The model under review builds one solid part; all positions refer to its coordinate system, in mm. Round coordinates to 2 decimals unless told otherwise and drop trailing zeros. Order: outer loops, then holes, each group sorted by start corner. A loop starts at its lowest first (then second) coordinate and runs counter-clockwise, first axis right, second up.
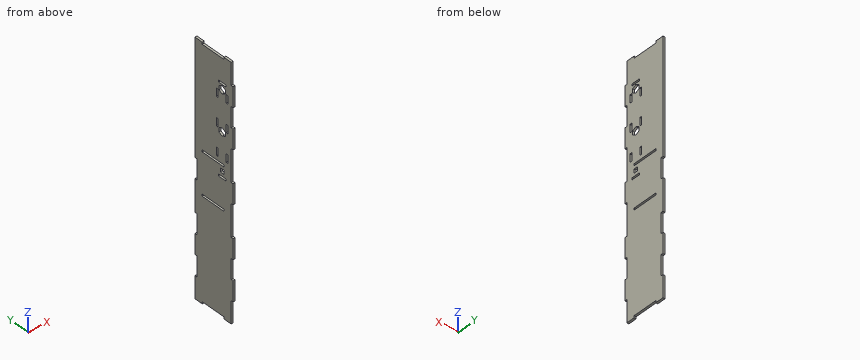
Autodesk Inventor part; units mm, degrees
ref_plane "YZ Plane" through (0, 0, 0) normal (1, 0, 0) x (0, 1, 0)
ref_plane "XZ Plane" through (0, 0, 0) normal (0, 1, 0) x (-1, 0, 0)
ref_plane "XY Plane" through (0, 0, 0) normal (0, 0, 1) x (1, 0, 0)
sketch "Sketch1" plane through (0, 0, 0) normal (1, 0, 0) x (0, 1, 0)
  line L0 (-50, 50) -> (50, 50)
  line L1 (50, 50) -> (50, -50)
  line L2 (50, -50) -> (-50, -50)
  line L3 (-50, -50) -> (-50, 50)
  line L4 (-50, 50) -> (50, -50) construction
  line L5 (50, 50) -> (-50, -50) construction
  line L6 (50, 50) -> (-50, 50)
  line L7 (-50, 50) -> (-50, 310)
  line L8 (-50, 310) -> (50, 310)
  line L9 (50, 310) -> (50, 50)
  line L10 (50, -50) -> (-50, -50)
  line L11 (-50, -50) -> (-50, -310)
  line L12 (-50, -310) -> (50, -310)
  line L13 (50, -310) -> (50, -50)
  line L14 (-50, 255) -> (-55, 255)
  line L15 (-55, 255) -> (-55, 205)
  line L16 (-55, 205) -> (-50, 205)
  line L17 (-50, 205) -> (-50, 255)
  line L18 (-50, 155) -> (-55, 155)
  line L19 (-55, 155) -> (-55, 105)
  line L20 (-55, 105) -> (-50, 105)
  line L21 (-50, 105) -> (-50, 155)
  line L22 (-50, 25) -> (-55, 25)
  line L23 (-55, 25) -> (-55, -25)
  line L24 (-55, -25) -> (-50, -25)
  line L25 (-50, -25) -> (-50, 25)
  line L26 (-50, -105) -> (-55, -105)
  line L27 (-55, -105) -> (-55, -155)
  line L28 (-55, -155) -> (-50, -155)
  line L29 (-50, -155) -> (-50, -105)
  line L30 (-50, -205) -> (-55, -205)
  line L31 (-55, -205) -> (-55, -255)
  line L32 (-55, -255) -> (-50, -255)
  line L33 (-50, -255) -> (-50, -205)
  line L34 (50, 310) -> (30, 310)
  line L35 (50, 305) -> (50, 310)
  line L36 (-50, 310) -> (-30, 310)
  line L37 (-50, 305) -> (-50, 310)
  line L38 (30, 50) -> (-30, 50)
  line L39 (-30, 50) -> (-30, 55)
  line L40 (-30, 55) -> (30, 55)
  line L41 (30, 55) -> (30, 50)
  line L42 (30, -50) -> (-21.1124, -50)
  line L43 (50, 0) -> (-50, 0) construction
  line L44 (-30, -50) -> (-30, -55)
  line L45 (-30, -55) -> (30, -55)
  line L46 (30, -55) -> (30, -50)
  line L47 (30, 310) -> (-30, 310)
  line L48 (-30, 310) -> (-30, 305)
  line L49 (-30, 305) -> (30, 305)
  line L50 (30, 305) -> (30, 310)
  line L51 (-30, -310) -> (-30, -305)
  line L52 (-30, -305) -> (30, -305)
  line L53 (30, -305) -> (30, -310)
  line L54 (50, 25) -> (45, 25)
  line L55 (45, 25) -> (45, -25)
  line L56 (45, -25) -> (50, -25)
  line L57 (50, -25) -> (50, 25)
  line L58 (50, -105) -> (45, -105)
  line L59 (45, -105) -> (45, -155)
  line L60 (45, -155) -> (50, -155)
  line L61 (50, -155) -> (50, -105)
  line L62 (50, -205) -> (45, -205)
  line L63 (45, -205) -> (45, -255)
  line L64 (45, -255) -> (50, -255)
  line L65 (50, -255) -> (50, -205)
  line L66 (-33.6603, 235) -> (-25, 240)
  line L67 (-25, 240) -> (-16.3397, 235)
  line L68 (-16.3397, 235) -> (-16.3397, 225)
  line L69 (-16.3397, 225) -> (-25, 220)
  line L70 (-25, 220) -> (-33.6603, 225)
  line L71 (-33.6603, 225) -> (-33.6603, 235)
  line L72 (-33.6603, 135) -> (-25, 140)
  line L73 (-25, 140) -> (-16.3397, 135)
  line L74 (-16.3397, 135) -> (-16.3397, 125)
  line L75 (-16.3397, 125) -> (-25, 120)
  line L76 (-25, 120) -> (-33.6603, 125)
  line L77 (-33.6603, 125) -> (-33.6603, 135)
  line L78 (-8.75, 225) -> (-13.75, 225)
  line L79 (-13.75, 225) -> (-13.75, 205)
  line L80 (-13.75, 205) -> (-8.75, 205)
  line L81 (-8.75, 205) -> (-8.75, 225)
  line L82 (-13.75, 135) -> (-8.75, 135)
  line L83 (-8.75, 135) -> (-8.75, 155)
  line L84 (-8.75, 155) -> (-13.75, 155)
  line L85 (-13.75, 155) -> (-13.75, 135)
  line L86 (-13.75, 85) -> (-8.75, 85)
  line L87 (-8.75, 85) -> (-8.75, 65)
  line L88 (-8.75, 65) -> (-13.75, 65)
  line L89 (-13.75, 65) -> (-13.75, 85)
  line L90 (-15, 242.5) -> (-35, 242.5)
  line L91 (-35, 242.5) -> (-35, 247.5)
  line L92 (-35, 247.5) -> (-15, 247.5)
  line L93 (-15, 247.5) -> (-15, 242.5)
  line L94 (-25, 361.7934) -> (-25, -98.4217) construction
  line L95 (-41.25, 65) -> (-36.25, 65)
  line L96 (-36.25, 65) -> (-36.25, 85)
  line L97 (-36.25, 85) -> (-41.25, 85)
  line L98 (-41.25, 85) -> (-41.25, 65)
  line L99 (-36.25, 135) -> (-41.25, 135)
  line L100 (-36.25, 155) -> (-36.25, 135)
  line L101 (-41.25, 135) -> (-41.25, 155)
  line L102 (-41.25, 155) -> (-36.25, 155)
  line L103 (-36.25, 205) -> (-41.25, 205)
  line L104 (-36.25, 225) -> (-36.25, 205)
  line L105 (-41.25, 225) -> (-36.25, 225)
  line L106 (-41.25, 205) -> (-41.25, 225)
  line L107 (-35, 20) -> (-15, 20)
  line L108 (-15, 20) -> (-15, 25)
  line L109 (-15, 25) -> (-35, 25)
  line L110 (-35, 25) -> (-35, 20)
  line L111 (-20, 42.5) -> (-30, 42.5)
  line L112 (-30, 42.5) -> (-30, 32.5)
  line L113 (-30, 32.5) -> (-20, 32.5)
  line L114 (-20, 32.5) -> (-20, 42.5)
  point P0 (0, 0)
  point P1 (-52.5, 155)
  point P2 (-52.5, 205)
  point P3 (-50, 205)
  point P4 (-50, 105)
  point P5 (-50, -155)
  point P6 (-50, -255)
  point P7 (30, -50)
  point P8 (-30, -50)
  point P9 (30, 50)
  point P10 (30, 307.5)
  point P11 (-30, -310)
  point P12 (30, 310)
  point P13 (-30, 310)
  point P14 (50, -25)
  point P15 (50, -255)
  point P16 (50, -155)
  point P17 (-25, 230)
  point P18 (-25, 130)
  point P19 (-13.75, 145)
  point P20 (-15, 245)
  point P21 (-36.25, 145)
  point P22 (-20, 37.5)
  dimension "d0" = 100
  dimension "d1" = 260
  dimension "d2" = 100
  dimension "d3" = 260
  dimension "d4" = 50
  dimension "d5" = 50
  dimension "d6" = 50
  dimension "d7" = 50
  dimension "d8" = 50
  dimension "d9" = 55
  dimension "d10" = 50
  dimension "d11" = 25
  dimension "d12" = 55
  dimension "d13" = 50
  dimension "d14" = 5
  dimension "d20" = 5
  dimension "d21" = 5
  dimension "d23" = 20
  dimension "d24" = 50
  dimension "d25" = 5
  dimension "d26" = 20
  dimension "d27" = 10
  dimension "d28" = 25
  dimension "d29" = 16.3397
  dimension "d30" = 25
  dimension "d31" = 10
  dimension "d32" = 25
  dimension "d33" = 16.3397
  dimension "d34" = 25
  dimension "d38" = 20
  dimension "d40" = 5
  dimension "d41" = 20
  dimension "d42" = 5
  dimension "d45" = 20
  dimension "d46" = 5
  dimension "d48" = 20
  dimension "d49" = 5
  dimension "d51" = 25
  dimension "d52" = 50
  dimension "d53" = 50
  dimension "d54" = 11.25
  dimension "d55" = 12.5
  dimension "d56" = 10
  dimension "d57" = 20
  dimension "d58" = 5
  dimension "d59" = 40
  dimension "d60" = 10
  dimension "d61" = 10
  dimension "d62" = 10
  dimension "d63" = 5
  dimension "d64" = 7.5
extrude "Extrusion1" add sketch "Sketch1" along normal blind 5 contours L7 L8 L48 L49 L50 L9 L0 L41 L40 L39 | L0 L1 L54 L55 L56 L2 L3 | L3 L24 L23 L22 | L20 L19 L18 L7 | L2 L44 L45 L46 L13 L58 L59 L60 L62 L63 L64 L12 L53 L52 L51 L11 | L16 L15 L14 L7 | L11 L28 L27 L26 | L11 L32 L31 L30
equation "\"BendRadius\" = Thickness"
equation "\"BendReliefWidth\" = Thickness"
equation "\"BendReliefDepth\" = 0.5 * Thickness"
equation "\"CornerReliefSize\" = 4 * Thickness"
equation "\"MinimumRemnant\" = 2 * Thickness"
equation "\"TransitionRadius\" = BendRadius"
equation "\"JacobiRadiusSize\" = BendRadius"
equation "\"GapSize\" = Thickness"
properties part number "Lat3" material "Wood (Cherry)"
(1) We need section B-B (x = 1.85). Count the separate pieces of the cut face and the enclosed holes in it, and give its area (3 significant figures).
(2) Clearance check with flat-ended pins moving along their axes: P1, Ø1.5, axis at x = 2, y = -53, coming from the -Z side; P2, Ø1.5, axis at x = 2, y = -6.5, coming from the +Z side; P3, Ø1.5, axis at x = 2, z = 293.5, coming from the -Y side. State where each tip first meets the part, or that it passes through.
(3) We need section C-C (z = -179.5). Give the boundary of the cut face in (x, y).
(4) We need section A-A (y = 18.5). Give the boundary of the cut face in (x, z).
(5) To check wall thickness, follow L1, parallel to Z at x = 1.1, y = -4.5; L2, parallel to Y at x = 3.05, z = 84; L3, parallel to Y at x = 1.15, z = -273. State the ranges of each line that lie inside material, in increasing order.
Verdict:
1. separate pieces: 1
1. enclosed holes: 13
1. area: 59,900 mm2
2. P1: stops at z = -255
2. P2: stops at z = 305
2. P3: stops at y = -50
3. outline: (0, -50) - (5, -50) - (5, 50) - (0, 50) - close
4. outline: (0, -305) - (5, -305) - (5, -55) - (0, -55) - close; (0, -50) - (5, -50) - (5, 50) - (0, 50) - close; (0, 55) - (5, 55) - (5, 305) - (0, 305) - close
5. L1: z = -305 to -55, -50 to 50, 55 to 305
5. L2: y = -50 to -41.25, -36.25 to -13.75, -8.75 to 50
5. L3: y = -50 to 50
